Autodesk Inventor part; units mm, degrees
ref_plane "YZ Plane" through (0, 0, 0) normal (1, 0, 0) x (0, 1, 0)
ref_plane "XZ Plane" through (0, 0, 0) normal (0, 1, 0) x (-1, 0, 0)
ref_plane "XY Plane" through (0, 0, 0) normal (0, 0, 1) x (1, 0, 0)
sketch "Sketch1" plane through (0, 0, 0) normal (0, 1, 0) x (-1, 0, 0)
  line L0 (0, 0) -> (-142.24, 0)
  line L1 (-142.24, 0) -> (-142.24, -24.765)
  line L2 (-142.24, -24.765) -> (0, -24.765)
  line L3 (0, -24.765) -> (0, 0)
  dimension "d0" = 142.24
  dimension "d1" = 24.765
extrude "Extrusion1" add sketch "Sketch1" along normal blind 50.165
fillet "Fillet1" radius 12.3698 2 edges at (0, 25.0825, 0) (0, 25.0825, -24.765)
fillet "Fillet2" radius 1.27 14 edges at (3.623, 50.165, -3.623) (0, 50.165, -12.3825) (3.623, 50.165, -21.142) (77.3049, 50.165, -24.765) (77.3049, 50.165, 0) (142.24, 50.165, -12.3825) (142.24, 25.0825, 0) (142.24, 25.0825, -24.765) (142.24, 0, -12.3825) (3.623, 0, -21.142) (0, 0, -12.3825) (3.623, 0, -3.623) (77.3049, 0, 0) (77.3049, 0, -24.765)
sketch "Sketch2" plane through (0, 50.165, 0) normal (0, 1, 0) x (1, 0, 0)
  line L0 (12.3698, 23.495) -> (140.97, 23.495)
  arc A0 (12.3698, 23.495) -> (1.27, 12.3952) centre (12.3698, 12.3952) ccw
  line L1 (1.27, 12.3698) -> (1.27, 12.3952)
  arc A1 (1.27, 12.3698) -> (12.3698, 1.27) centre (12.3698, 12.3698) ccw
  line L2 (140.97, 1.27) -> (12.3698, 1.27)
  line L3 (140.97, 23.495) -> (140.97, 1.27)
  line L4 (12.3698, 12.3698) -> (5.7707, 16.1798)
  line L5 (12.3698, 12.3698) -> (19.9898, 12.3698) construction
  line L6 (12.3698, 12.3698) -> (5.7707, 8.5598)
  line L7 (12.3698, 12.3698) -> (19.9898, 12.3698) construction
  circle A2 centre (5.7707, 8.5598) radius 3.175
  circle A3 centre (5.7707, 16.1798) radius 3.175
  point P0 (0, 0)
  dimension "d6" = 7.62
  dimension "d7" = 150
  dimension "d8" = 7.62
  dimension "d9" = 150
  dimension "d10" = 6.35
  dimension "d11" = 6.35
extrude "Extrusion2" add sketch "Sketch2" along normal blind 12.7 contours A3 | A2
properties part number "Battery"
CAD build for the part. Positions are in the model's coordinates, mm. A direction names the side the tool comes from. Give positions to 0.01 mm unless a question says otherwise; leave off trailing zeros. Order: outer loops, then holes, each group sorted by start corner. A loop starts at its lowest first (then second) coordinate and runs counter-clockwise, first axis right, second up.
(1) Flat gauge pin, fed straight in: pin 1 (2 mm diameter, centred on y = 16, z = -10, fed in from -X). Where does the tip first touch, or does it go through?
(2) Tool access for faces 1 (the cylindrical face through (7.236, 56.426, -11.377)), 2 (the flat face through (72, 0, -12)): list every direction of +Z, -Z, +X, -X, +Y, -Y with a clear straight run to the whole face (end or side of a thin tool).
(3) Saw through at A-A, the plane x = 27. Give the cut face in (y, z) (3 decimals).
(4) Saw through at C-C, the plane y = 53.5. Give the cut face in (x, z) (3 decimals).
(5) Mould opens along Z. For faces 3 (the cylindrical face through (3.527, 25.416, -3.72)), 4 (the cylindrical face through (5.36, 56.43, -13.03)), 5 (the flat face through (6, 62.865, -9)) say: released by +Z, released by -Z, zero draft, split by the parting line, or undercut.
(6) Drill centre lines: L1, parallel to Y at x = 116, z = -9.75 (3 decimals); L2, parallel to Y at x = 99, z = -0.75; L3, parallel to X at y = 19, z = -9. Where is each one in solid material? Low to high.
(7) Saw through at B-B, the plane y = 4. Give the cut face in (x, z) (3 decimals).
Results found:
1. pin 1: stops at x = 0.08
2. face 1: +Y
2. face 2: +Z, -Z, +X, -X, -Y
3. outline: (0, -23.495) arc R1.27 ccw to (1.27, -24.765) - (48.895, -24.765) arc R1.27 ccw to (50.165, -23.495) - (50.165, -1.27) arc R1.27 ccw to (48.895, 0) - (1.27, 0) arc R1.27 ccw to (0, -1.27) - close
4. outline: circle Ø6.35 at (5.771, -16.18); circle Ø6.35 at (5.771, -8.56)
5. face 3: released by +Z
5. face 4: undercut
5. face 5: zero draft
6. L1: y = 0 to 50.165
6. L2: y = 0.11 to 50.05
6. L3: x = 0.47 to 142.24
7. outline: (0, -12.395) arc R12.37 ccw to (12.37, -24.765) - (140.97, -24.765) arc R1.27 ccw to (142.24, -23.495) - (142.24, -1.27) arc R1.27 ccw to (140.97, 0) - (12.37, 0) arc R12.37 ccw to (0, -12.37) - close
